Here's the drawing with two shaded views (mm, measured from the low corner). I have some questions. A direction names the side the tool comes from. Round coordinates to 2 decimals unless told otherwise and drop trailing zeros. Loops run counter-clockwise (first coordinate to the right, second up) from the corner with the lowest first, then second, coordinate; pieces in that order, holes last. Notation, with made-up numbers: M 64,1.25 L 92,1.25 A3 cw 92,5.25 Z; hole C -12.75,10.25 d9. An arc over 180 degrees is marked long. One line per item, written item: value. Start each with the question number.
Q1. Thinking about a two-plate mould opening in X: for the marked faces 3, 4 and 5, which applies, released by +X, released by -X, zero draft, split by the parting line, or undercut?
Q2. I'm going to push flat-ended pins straight in: pin 1 Ø19 at (x, z) = (33, 19) entering from -Y; pin 2 Ø2.5 at (y, z) = (40, 21.5) entering from +X; pin 3 Ø3.5 at (y, z) = (39, 30) entering from -X. Where does each tip first touch, or does it pass through?
Q3. Please list where these lines run through material, in increasing order: line 1 along X through (y, z) = (33, 2.5) (3 decimals); line 2 along Z through (x, y) = (3, 9); line 3 along Y through (x, z) = (44.5, 5) (3 decimals).
Q4. Imagine slicing it at A-A (y = 34). Please give me the cut outline in (x, z) (3 decimals), then the cut area to 4 significant figures.
Q5. Imagine slicing it at C-C (x = 53). Please give me the cut outline in (y, z) (3 decimals), then the cut area to 3 significant figures.
Q6. Imagine slicing it at B-B (z = 11.5). Please give me the cut outline in (x, y) (3 decimals).
Q7. Which directions (+Z, -Z, +X, -X, +Y, -Y) give clear straight access to the entire face, cutting with the end or side of a thin tool? Please do the marked faces 1 and 2.
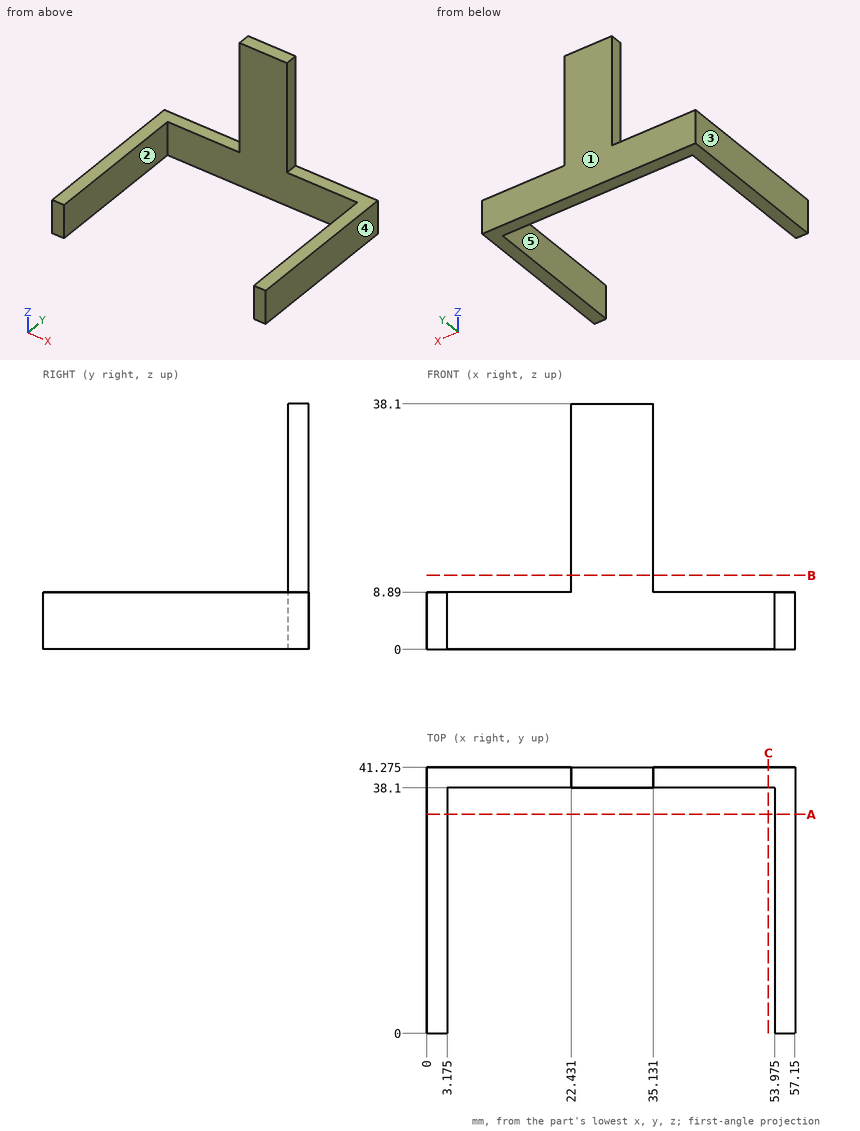
Report:
1. face 3: released by -X
1. face 4: released by +X
1. face 5: undercut
2. pin 1: stops at y = 38.1
2. pin 2: stops at x = 35.13
2. pin 3: stops at x = 22.43
3. line 1: x = 0 to 3.175, 53.975 to 57.15
3. line 2: z = 0 to 8.89
3. line 3: y = 38.1 to 41.275
4. outline: M 0,0 L 3.175,0 L 3.175,8.89 L 0,8.89 Z; M 53.975,0 L 57.15,0 L 57.15,8.89 L 53.975,8.89 Z
4. area: 56.45 mm²
5. outline: M 38.1,0 L 41.275,0 L 41.275,8.89 L 38.1,8.89 Z
5. area: 28.2 mm²
6. outline: M 22.431,38.1 L 35.131,38.1 L 35.131,41.275 L 22.431,41.275 Z
7. face 1: +Z, -Z, +X, -X, +Y
7. face 2: +Z, -Z, -Y
